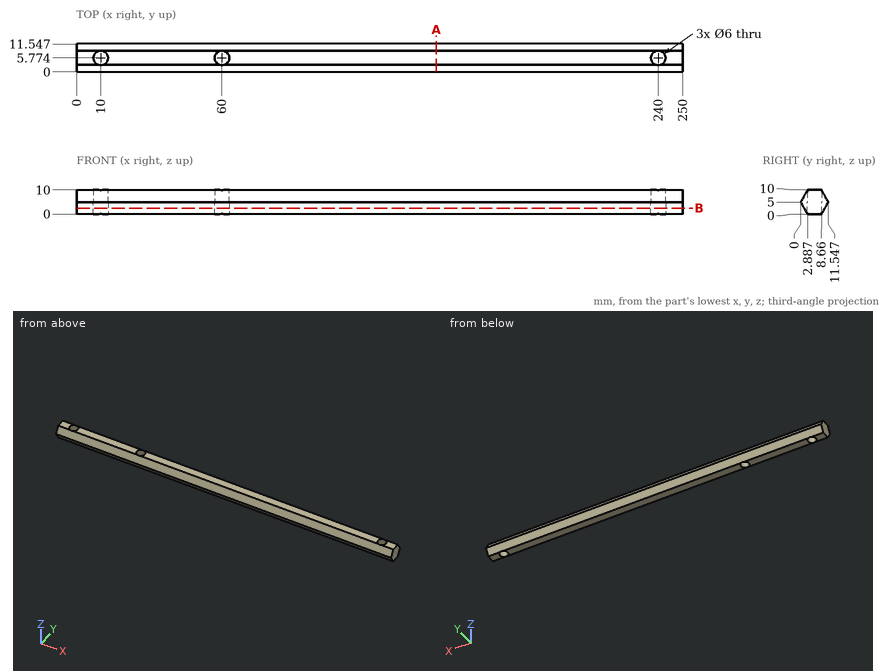
Answer from the drawing. Dimensions are ordinates in mm from the lowest x, y and z of the part. Give positions to 0.01 mm unless a question says otherwise; leave off trailing zeros. Order: outer loops, then holes, each group sorted by start corner. A loop starts at its lowest first (then second) coordinate and runs counter-clockwise, first axis right, second up. Notation, with made-up numbers: (11.5, 70.5) - (59.5, 70.5) arc R27 ccw to (59.5, 87.5) - close; hole circle Ø7 at (-39, 18). An arc over 180 degrees is marked (long way). One line per item, written item: value. Start each with the question number.
1. This flat-tipped pin is pushed along its axis until it touches: pin 1 Ø6 at (x, z) = (53.5, 6) entering from -Y. Where does it stop, or does it pass through?
2. Section A-A, the plane x = 148.5 is taken. Write down the section's boundary in (y, z), then the cut area to 3 significant figures.
3. Consider line 1 (X direction, y = 5.25, z = 3) (1 decimal); line 2 (X direction, y = 6.5, z = 3.5); line 3 (Y direction, x = 10, z = 7.5) (1 decimal). Determine where each line is inside the solid, lowest interval first.
4. Section B-B, the plane z = 2.5 is taken. Write down the section's boundary in (x, y).
Filled sheet:
1. pin 1: y = 0
2. outline: (0, 5) - (2.89, 0) - (8.66, 0) - (11.55, 5) - (8.66, 10) - (2.89, 10) - close
2. area: 86.6 mm²
3. line 1: 0 to 7, 13 to 57, 63 to 237, 243 to 250
3. line 2: 0 to 7.09, 12.91 to 57.09, 62.91 to 237.09, 242.91 to 250
3. line 3: 1.4 to 2.8, 8.8 to 10.1
4. outline: (0, 1.44) - (250, 1.44) - (250, 10.1) - (0, 10.1) - close; hole circle Ø6 at (10, 5.77); hole circle Ø6 at (60, 5.77); hole circle Ø6 at (240, 5.77)
